Could you check a few things on this model? Use its own coordinates, in mm. Round coordinates to 2 decimals unless told otherwise and drop trailing zeros. Loops run counter-clockwise (first coordinate to the right, second up) from the corner with the lowest first, then second, coordinate; pieces in that order, holes last. Notation, with made-up numbers: (45, 29) - (73, 29) arc R17 ccw to (73, 51) - close; hole circle Ø6 at (-14, -36). An arc over 180 degrees is marked (long way). Answer as CSV lines item,"result". Start each with the question number.
1) Suppose I cut it at C-C, the plane z = 4. Count the separate pieces of the cut face and the enclosed holes in it, then the cut area to 3 significant figures.
2) I'm going to push flat-ended pins straight in: pin 1 Ø1 at (x, z) = (72, 4.5) entering from +Y; pin 2 Ø4 at (x, z) = (-22.5, 5) entering from +Y; pin 3 Ø5 at (y, z) = (104.5, 4.5) entering from +X. Where does each tip first touch, or does it pass through?
3) Suppose I cut it at A-A, the plane x = 12.5. Write out the boundary of the cut face in (y, z), then the cut area to 4 significant figures.
4) Please list where these lines run through material, in increasing order: line 1 along Y through (x, z) = (-57, 7.75); line 2 along X through (y, z) = (-21, 6.75); line 3 along X through (y, z) = (97, 8.25).
5) Suppose I cut it at B-B, the plane y = 6.5. Write out the boundary of the cut face in (x, z), then the cut area to 3 significant figures.
```python
from build123d import *

# Parameters (mm, degrees)
BOSS_EXTRU_1_DEPTH = 8.5


with BuildPart() as part:
    # Esquisse1 → Boss.-Extru.1 (new body)
    with BuildSketch(Plane.XY):
        Polygon((-76.753762562, 40.085106383), (2.011353671, 40.085106383), (50.71612997, 40.085106383), (151.689760112, 98.382258927), (214.4831558, 115.207698591), (229.494660416, 59.184000666), (174.076924484, 44.334863077), (66.257183131, -17.914893617), (-98.698564415, -17.914893617), (-98.698564415, 40.655573641), (-94.860830925, 40.655573641), (-92.861789188, 40.655573641), (-92.861789188, 48.636078378), (-92.861789188, 50.298812036), (-92.861789188, 51.585106383), (-94.860830925, 51.585106383), (-96.789296468, 51.585106383), (-103.253762562, 45.120640289), (-103.253762562, 35.79522772), (-103.253762562, -22.950427523), (-96.789296468, -29.414893617), (63.997857106, -29.414893617), (73.963816863, -26.744522748), (178.515758799, 33.618569072), (237.335031683, 49.379145741), (241.906099495, 57.296467436), (230.508864659, 99.83152691), (225.851857518, 117.211714172), (224.321712805, 123.047343228), (216.426306891, 127.634040432), (210.540810955, 126.057026548), (147.250925797, 109.098552931), (51.669750275, 53.914735514), (42.975455994, 51.585106383), (-75.988646329, 51.585106383), (-76.753762562, 51.585106383), (-76.753762562, 50.298812036), (-76.753762562, 49.585106383), (-76.753762562, 48.636078378), align=None)
        Polygon((-95.09515421, -19.181421764), (-93.057202321, -21.118529255), (-93.715810673, -23.852001108), (-96.412370914, -24.64836547), (-98.450322803, -22.71125798), (-97.791714451, -19.977786126), align=None, mode=Mode.SUBTRACT)
        Polygon((67.767414571, -18.119374886), (69.755583746, -20.107544061), (69.027863321, -22.82343366), (66.311973721, -23.551154085), (64.323804547, -21.56298491), (65.051524972, -18.847095311), align=None, mode=Mode.SUBTRACT)
        Polygon((-93.318762562, 45.490954288), (-93.318762562, 42.679258478), (-95.753762562, 41.273410572), (-98.188762562, 42.679258478), (-98.188762562, 45.490954288), (-95.753762562, 46.896802194), align=None, mode=Mode.SUBTRACT)
        Polygon((-66.988646329, 46.896802194), (-64.553646329, 45.490954288), (-64.553646329, 42.679258478), (-66.988646329, 41.273410572), (-69.423646329, 42.679258478), (-69.423646329, 45.490954288), align=None, mode=Mode.SUBTRACT)
        Polygon((51.366225237, 47.372350111), (51.931744927, 44.618113227), (49.829265662, 42.751240367), (47.161266708, 43.638604392), (46.595747018, 46.392841276), (48.698226283, 48.259714136), align=None, mode=Mode.SUBTRACT)
        Polygon((176.099626255, 43.341034088), (178.27036991, 41.553995947), (177.808121311, 38.780557726), (175.175129056, 37.794157645), (173.004385401, 39.581195786), (173.466634, 42.354634007), align=None, mode=Mode.SUBTRACT)
        Polygon((235.851309069, 58.804459007), (237.257156975, 56.369459007), (235.851309069, 53.934459007), (233.039613258, 53.934459007), (231.633765353, 56.369459007), (233.039613258, 58.804459007), align=None, mode=Mode.SUBTRACT)
        Polygon((150.436891261, 104.94434728), (152.703485209, 103.280560873), (152.395900888, 100.48573973), (149.821722619, 99.354704995), (147.555128671, 101.018491402), (147.862712992, 103.813312544), align=None, mode=Mode.SUBTRACT)
        Polygon((219.824270363, 121.480626406), (219.771686266, 118.66942235), (217.310820089, 117.309359486), (214.90253801, 118.760500678), (214.955122108, 121.571704735), (217.415988284, 122.931767598), align=None, mode=Mode.SUBTRACT)
    extrude(amount=BOSS_EXTRU_1_DEPTH)


solid = part.part
```
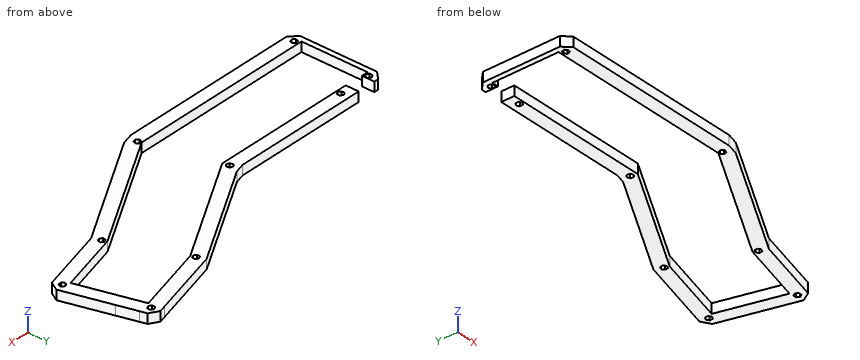
Filled sheet:
1,separate pieces,"1"
1,enclosed holes,"9"
1,area,"8,640 mm²"
2,pin 1,"y = 65.94"
2,pin 2,"y = 51.59"
2,pin 3,"x = 229.93"
3,outline,"(-29.41, 0) - (-17.91, 0) - (-17.91, 8.5) - (-29.41, 8.5) - close; (40.09, 0) - (51.59, 0) - (51.59, 8.5) - (40.09, 8.5) - close"
3,area,"195.5 mm²"
4,line 1,"-29.41 to -17.91, 40.09 to 51.59"
4,line 2,"-103.25 to -98.04, -93.18 to 64.47, 69.52 to 83.91"
4,line 3,"126.3 to 149.3, 219.36 to 231.27"
5,outline,"(-103.25, 0) - (-98.7, 0) - (-98.7, 8.5) - (-103.25, 8.5) - close; (108.55, 0) - (131.55, 0) - (131.55, 8.5) - (108.55, 8.5) - close"
5,area,"234 mm²"
